Can you work these out from the model? Positions are in its coordinate system, mm. Face numbers are marked on the shaded views. Round coordinates to 2 decimals unless told otherwise and drop trailing zeros. Write each loop counter-clockwise with the first axis right and the second up, starting at its lowest first coordinate (ties: lowest second). Pieces come first, ordered by that corner, then holes. Notation, with made-up numbers: (13, -23) - (33, -23) arc R21 cw to (33, -16) - close; hole circle Ø11 at (-6, 49.5). An arc over 180 degrees is marked (long way). One line per item, written item: value. Start each with the question number.
(1) I want a section at A-A on z = 10. Give the number of separate pieces and of enclosed holes in the cut face, plus the area to 3 significant figures.
(2) I want a section at C-C on x = -0.5. List the corners of the cut face in (y, z) for me, plus the area to 3 significant figures.
(3) I'm going to push flat-ended pins straight in: pin 1 Ø5 at (x, y) = (0, 27.6) entering from -Z; pin 2 Ø1.5 at (x, z) = (-2.5, 7) entering from -Y; pin 3 Ø8 at (x, z) = (23.5, -10) entering from +Y; pin 4 Ø8 at (x, z) = (8, 9.5) entering from +Y. Where does each tip first touch, or does it pass through?
(4) If I drill on L1, parallel to Y at x = 0, z = -18; L2, parallel to X at y = -2, z = -18.5; L3, parallel to Y at x = 3.5, z = 14.5, over which ranges is the centre line in solid material (lowest first)? Write a range as from..to.
(5) I want a section at B-B on y = -27.6. List the corners of the cut face in (x, z) for me, plus the area to 3 significant figures.
(6) Thinking about a two-plate mould opening in Y: for the marked faces 1 and 2, which applies, +Y half, -Y half, draft (parallel to the pull), parting line (faces both ways), or undercut?
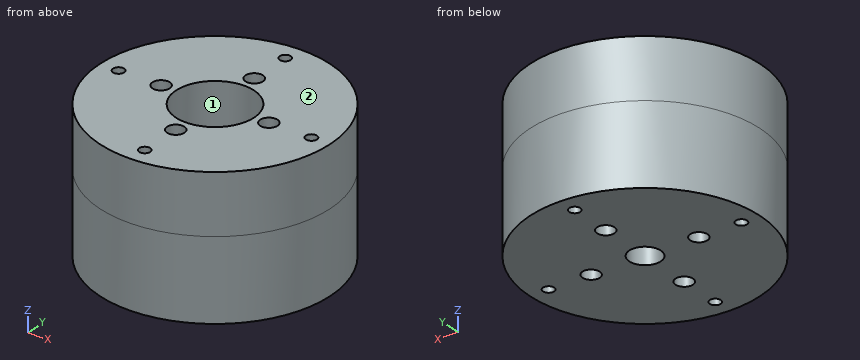
from build123d import *

# Parameters (mm, degrees)
F0_R     = 33
F0_R_2   = 11.2
F1_DEPTH = 23
F2_R     = 4.5
F3_DEPTH = 23.001
F4_DEPTH = 17
F5_R     = 2.5
F5_R_2   = 1.6
F6_DEPTH = 40.001


with BuildPart() as f1:
    # F0 (on Top) → F1 (new body)
    with BuildSketch(Plane.XY):
        Circle(F0_R)
        Circle(F0_R_2, mode=Mode.SUBTRACT)
        Circle(F0_R_2)
    extrude(amount=-F1_DEPTH)

    # F2 (on face) → F3 (cut, through all)
    with BuildSketch(Plane.XY):
        Circle(F2_R)
    extrude(amount=-F3_DEPTH, mode=Mode.SUBTRACT)

    # F0 (on Top) → F4 (join)
    with BuildSketch(Plane.XY):
        Circle(F0_R)
        Circle(F0_R_2, mode=Mode.SUBTRACT)
    extrude(amount=F4_DEPTH)

    # F5 (on face) → F6 (cut, through all)
    with BuildSketch(Plane.XY.offset(17)):
        with Locations((15.42, 0)):
            Circle(F5_R)
        with Locations((0, -15.42)):
            Circle(F5_R)
        with Locations((0, 15.42)):
            Circle(F5_R)
        with Locations((-15.42, 0)):
            Circle(F5_R)
        with Locations((27.6, 0)):
            Circle(F5_R_2)
        with Locations((0, 27.6)):
            Circle(F5_R_2)
        with Locations((0, -27.6)):
            Circle(F5_R_2)
        with Locations((-27.6, 0)):
            Circle(F5_R_2)
    extrude(amount=-F6_DEPTH, mode=Mode.SUBTRACT)


solid = f1.part
Established:
1. separate pieces: 1
1. enclosed holes: 9
1. area: 2,920 mm2
2. outline: (-33, -23) - (-29.12, -23) - (-29.12, 17) - (-33, 17) - close; (-26.08, -23) - (-17.87, -23) - (-17.87, 17) - (-26.08, 17) - close; (-12.97, -23) - (-4.47, -23) - (-4.47, 0) - (-11.19, 0) - (-11.19, 17) - (-12.97, 17) - close; (4.47, -23) - (12.97, -23) - (12.97, 17) - (11.19, 17) - (11.19, 0) - (4.47, 0) - close; (17.87, -23) - (26.08, -23) - (26.08, 17) - (17.87, 17) - close; (29.12, -23) - (33, -23) - (33, 17) - (29.12, 17) - close
2. area: 1,420 mm2
3. pin 1: z = -23
3. pin 2: y = -32.95
3. pin 3: y = 26.62
3. pin 4: y = 32.76
4. L1: -33..-29.2, -26..-17.92, -12.92..-4.5, 4.5..12.92, 17.92..26, 29.2..33
4. L2: -32.94..-16.92, -13.92..-4.03, 4.03..13.92, 16.92..32.94
4. L3: -32.81..-10.64, 10.64..32.81
5. outline: (-18.09, -23) - (-1.6, -23) - (-1.6, 17) - (-18.09, 17) - close; (1.6, -23) - (18.09, -23) - (18.09, 17) - (1.6, 17) - close
5. area: 1,320 mm2
6. face 1: undercut
6. face 2: draft
